Source: CAD feature listing. Evaluate the final solid. Frame: model axes, mm. Face numbers are marked on the shaded views. A direction names the side the tool comes from. Coordinates: 2 decimals unless noted, no trailing zeros. Loops run counter-clockwise (first coordinate to the right, second up) from the corner with the lowest first, then second, coordinate; pieces in that order, holes last. Notation, with made-up numbers: (71, 87.25) -> (82, 87.25) arc R6 ccw to (82, 96.25) -> close; hole circle Ø9 at (48.5, 78). An arc over 180 degrees is marked (long way). Answer as CSV lines item,"result".
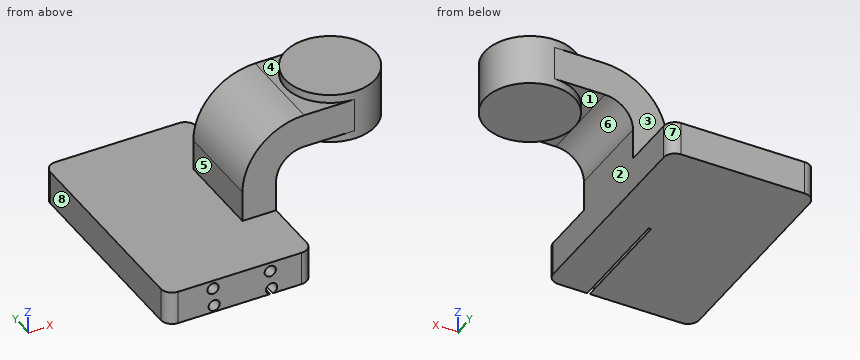
from build123d import *

# Parameters (mm, degrees)
F1_DEPTH = 63.5
F2_DEPTH = 25.4
F0_W     = 25.4
F0_H     = 19.05
F3_DEPTH = 25.4
F5_R     = 6.35
F7_D     = 6.35
F7_DEPTH = 63.501


with BuildPart() as f1:
    # F0 (on Front) → F1 (new body, symmetric)
    with BuildSketch(Plane.XZ):
        Polygon((41.275, -9.525), (41.275, 9.525), (22.225, 9.525), (-41.275, 9.525), (-41.275, -9.525), align=None)
    extrude(amount=F1_DEPTH, both=True)

    # F0 (on Front) → F2 (join, symmetric)
    with BuildSketch(Plane.XZ):
        with BuildLine():
            Line((22.225, 9.525), (41.275, 9.525))
            Line((41.275, 9.525), (41.275, 27.0002))
            ThreePointArc((41.275, 27.0002), (45.9246798487, 38.2255201513), (57.15, 42.8752))
            Line((57.15, 42.8752), (60.325, 42.8752))
            Line((60.325, 42.8752), (60.325, 61.9252))
            Line((60.325, 61.9252), (57.15, 61.9252))
            ThreePointArc((57.15, 61.9252), (32.4542956671, 51.6959043329), (22.225, 27.0002))
            Line((22.225, 27.0002), (22.225, 9.525))
        make_face()
    extrude(amount=F2_DEPTH, both=True)

    # F0 (on Front) → F3 (join, symmetric)
    with BuildSketch(Plane.XZ):
        with Locations((73.025, 52.4002)):
            Rectangle(F0_W, F0_H)
    extrude(amount=F3_DEPTH, both=True)

    # F0 (on Front) → F4 (revolve)
    with BuildSketch(Plane.XZ):
        Polygon((85.725, 61.9252), (85.725, 42.8752), (85.725, 38.1), (111.125, 38.1), (111.125, 66.675), (85.725, 66.675), align=None)
    revolve(axis=Axis((85.725, 0, 52.3875), (0, 0, 1)))

    # F5
    f5_edges = [f1.edges().sort_by_distance(p)[0] for p in [
        (-41.275, -63.5, 0),
        (41.275, -63.5, 0),
        (41.275, 63.5, 0),
        (-41.275, 63.5, 0),
    ]]
    fillet(f5_edges, radius=F5_R)

    # F7 (through all, one way)
    with BuildSketch(Plane(origin=(0, 0, 0), x_dir=(1, 0, 0), z_dir=(0, 1, 0))):
        with Locations((17.1776954085, -4.3224697001), (-15.1745518669, -4.7319913283), (-14.5602682605, 5.7108225301), (17.8943593055, 6.4274864271)):
            Circle(F7_D / 2)
    extrude(amount=-F7_DEPTH, mode=Mode.SUBTRACT)


solid = f1.part
(1) Material intervals for L1, parallel to X at y = -44.5, z = 4 (3 decimals); L2, parallel to X at y = 3.5, z = 8.5 (3 decimals); L3, parallel to Z at x = 39.5, y = 3.5 (3 decimals), sorted ascending. Write a range as [from, to].
Computed values:
L1,"[-41.275, -18.264], [-12.085, 14.019], [20.336, 41.275]"
L2,"[-41.275, 41.275]"
L3,"[-9.525, 57.137]"
(2) Draft query along X for the marked faces 6, 7 and 8. Return one class per face: released by +X, released by -X, zero draft, split by the parting line, or undercut.
Computed values:
face 6,"undercut"
face 7,"released by +X"
face 8,"released by -X"
(3) Cut plane A-A (y = -17). Return the cut outline in (x, z) (3 decimals).
Computed values:
outline,"(-41.275, -9.525) -> (17.197, -9.525) arc R3.175 cw (long way) to (18.592, -9.525) -> (41.275, -9.525) -> (41.275, 27) arc R15.875 cw to (57.15, 42.875) -> (66.853, 42.875) -> (66.853, 38.1) -> (104.597, 38.1) -> (104.597, 66.675) -> (66.853, 66.675) -> (66.853, 61.925) -> (57.15, 61.925) arc R34.925 ccw to (22.225, 27) -> (22.225, 9.525) -> (-41.275, 9.525) -> close; hole circle Ø6.35 at (-15.175, 4.732); hole circle Ø6.35 at (-14.56, -5.711); hole circle Ø6.35 at (17.178, 4.322)"
(4) Cut plane C-C (x = 25). Return the cut outline in (y, z) (3 decimals), then the cut area to 3 significant figures.
Computed values:
outline,"(-63.5, -9.525) -> (63.5, -9.525) -> (63.5, 9.525) -> (25.4, 9.525) -> (25.4, 40.643) -> (-25.4, 40.643) -> (-25.4, 9.525) -> (-63.5, 9.525) -> close"
area,"4,000 mm^2"
(5) Pin query (flat end, axial travel): pin 1 Ø1.9 at (x, z) = (-14.5, -5) entering from -Y; pin 2 Ø8 at (x, z) = (82.5, 37.5) entering from +Y; pin 3 Ø8.5 at (x, y) = (78, 8.5) entering from -Z. Return the tip coordinate at first contact, or that it passes through.
Computed values:
pin 1,"y = 0"
pin 2,"y = 25.4"
pin 3,"z = 38.1"
(6) Access query for the marked faces 1, 2, 3, 4 and 5. Directions: +Z, -Z, +X, -X, +Y, -Y. A direction counts if a zero-diameter tool reaches every point of the face in a straight line with its end or side. Return the directions, or none.
Computed values:
face 1,"-Z"
face 2,"-Z, +X, +Y, -Y"
face 3,"+Z, +X, -X, +Y"
face 4,"+Z, -X"
face 5,"+Z, -X, +Y, -Y"
(7) Cut plane D-D (y = 51.5). Return the cut outline in (x, z) (3 decimals), then the cut area to 3 significant figures.
Computed values:
outline,"(-41.275, -9.525) -> (41.275, -9.525) -> (41.275, 9.525) -> (-41.275, 9.525) -> close"
area,"1,570 mm^2"
(8) Cut plane B-B (y = 18.5). Return the cut outline in (x, z) (3 decimals), then the cut area to 3 significant figures.
Computed values:
outline,"(-41.275, -9.525) -> (41.275, -9.525) -> (41.275, 27) arc R15.875 cw to (57.15, 42.875) -> (68.321, 42.875) -> (68.321, 38.1) -> (103.129, 38.1) -> (103.129, 66.675) -> (68.321, 66.675) -> (68.321, 61.925) -> (57.15, 61.925) arc R34.925 ccw to (22.225, 27) -> (22.225, 9.525) -> (-41.275, 9.525) -> close"
area,"3,870 mm^2"
